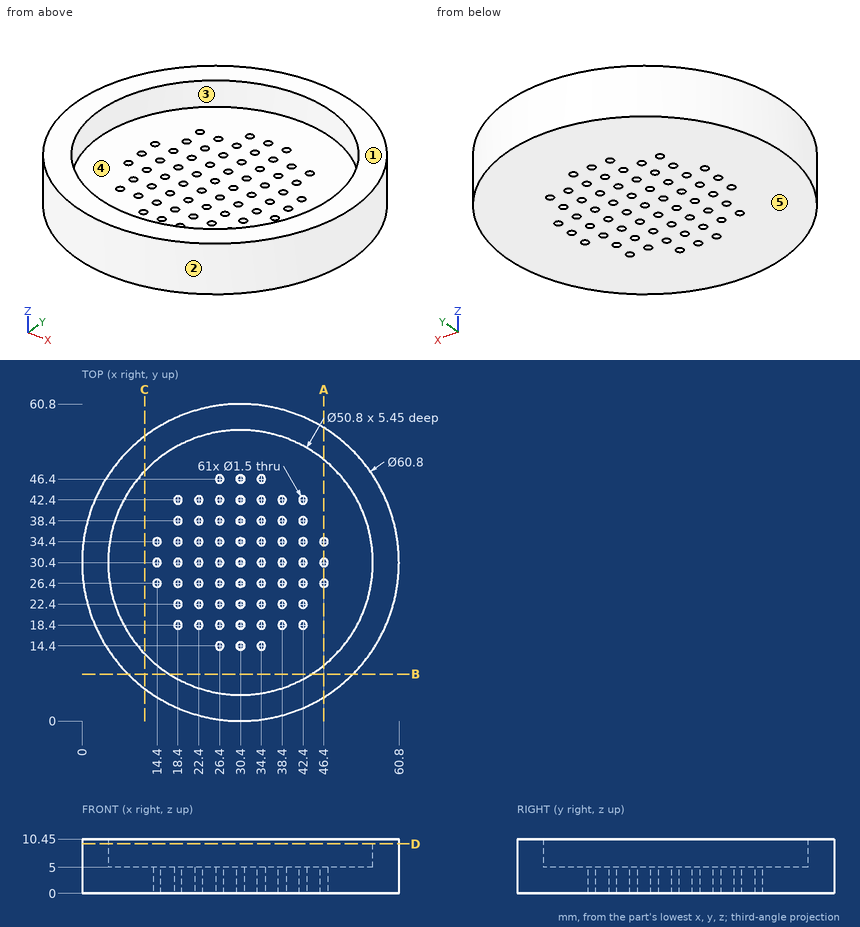
Geometry check sheet. Reference: drawing and pictorial views, mm from the part's lowest x, y, z. A direction names the side the tool comes from. Coordinates: 2 decimals unless noted, no trailing zeros. Order: outer loops, then holes, each group sorted by start corner. A loop starts at its lowest first (then second) coordinate and runs counter-clockwise, first axis right, second up.
Item 1: Depth check by flat-ended pin: pin 1 (2 mm diameter, centred on x = 38.4, y = 26.4, fed in from +Z); pin 2 (2 mm diameter, centred on x = 9, z = 8.5, fed in from +Y); pin 3 (1.5 mm diameter, centred on y = 36, z = 4, fed in from -X). Enter the tip coordinate at first touch or a pass-through.
Item 2: Section check A-A (x = 46.4). Enter the section's corners in (y, z), plus the area to 3 significant figures.
Item 3: Section check B-B (y = 9). Enter the section's corners in (x, z), plus the area to 3 significant figures.
Item 4: Section check C-C (x = 12). Enter the section's corners in (y, z), plus the area to 3 significant figures.
Item 5: Tool access check on the marked faces 4 and 5. Record the directions out of +Z, -Z, +X, -X, +Y, -Y that give a thin tool (end or side, any length) a straight path to the whole face; none if there is none.
Item 6: Section check D-D (z = 9.5). Enter the section's corners in (x, y).
Item 7: Mould release check, pull along X, two halves, no side actions. Record for the marked faces 1, 2 and 3: released by +X, released by -X, zero draft, split by the parting line, or undercut.
Item 8: Scan lines: line 1 along Y through (x, z) = (14.4, 2.7); line 2 along Y through (x, z) = (31, 7.25); line 3 along X through (y, z) = (9, 8.5). Record each from-to range of solid material in increasing order.
Check sheet entries:
1. pin 1: stops at z = 5
1. pin 2: stops at y = 52.94
1. pin 3: stops at x = 0.39
2. outline: (4.55, 0) - (25.65, 0) - (25.65, 5) - (10.67, 5) - (10.67, 10.45) - (4.55, 10.45) - close; (27.15, 0) - (29.65, 0) - (29.65, 5) - (27.15, 5) - close; (31.15, 0) - (33.65, 0) - (33.65, 5) - (31.15, 5) - close; (35.15, 0) - (56.25, 0) - (56.25, 10.45) - (50.13, 10.45) - (50.13, 5) - (35.15, 5) - close
2. area: 303 mm2
3. outline: (8.81, 0) - (51.99, 0) - (51.99, 10.45) - (44.08, 10.45) - (44.08, 5) - (16.72, 5) - (16.72, 10.45) - (8.81, 10.45) - close
3. area: 302 mm2
4. outline: (6.2, 0) - (54.6, 0) - (54.6, 10.45) - (47.91, 10.45) - (47.91, 5) - (12.89, 5) - (12.89, 10.45) - (6.2, 10.45) - close
4. area: 315 mm2
5. face 4: +Z
5. face 5: -Z, +X, -X, +Y, -Y
6. outline: circle Ø60.8 at (30.4, 30.4); hole circle Ø50.8 at (30.4, 30.4)
7. face 1: zero draft
7. face 2: split by the parting line
7. face 3: undercut
8. line 1: y = 4.55 to 25.65, 27.15 to 29.65, 31.15 to 33.65, 35.15 to 56.25
8. line 2: y = 0.01 to 5.01, 55.79 to 60.79
8. line 3: x = 8.81 to 16.72, 44.08 to 51.99
